Geometry: see drawing. Coordinates: mm, zero at the bounding-box minimum. A direction names the side the tool comes from. Give positions to 0.01 mm unless a question says otherwise; leave off trailing zeros. Order: outer loops, then holes, each group sorted by start corner. A loop starts at its lowest first (then second) coordinate and runs counter-clockwise, first axis right, second up. Notation, with made-up numbers: (82, 55.5) - (93, 55.5) arc R31 cw to (93, 87.5) - close; hole circle Ø11 at (-29.75, 64.25). An arc over 180 degrees is marked (long way). Put each result on its own line as item: value. Start each with the question number.
1. First-contact query: P1, Ø5.5, axis at y = 5, z = 32, coming from the -X side; P2, Ø5, axis at x = 19.85, z = 14, coming from the -Y side; P3, Ø3, axis at x = 52.25, y = 4.9, coming from the +Z side; P4, Ø10, axis at y = 14.5, z = 17.5, coming from the +X side. Flat tips, straight axial feed; report the tip coordinate or a pass-through.
2. Section B-B on x = 52.25. Return the cut outline in (y, z).
3. Section D-D on z = 14. Return the cut outline in (x, y), plus the area to 3 significant figures.
4. Set-up query: the marked faces 4, 5, 6, 7 and 8. Return all of +Z, -Z, +X, -X, +Y, -Y with unobstructed straight access to the full face (end or side cutting, diameter ignored); none if empty.
5. Section C-C on x = 19.85. Return the cut outline in (y, z), plus the area to 3 significant figures.
6. Ray query, line 1 along Y through (x, z) = (52.25, 27.75); line 2 along Z through (x, y) = (19.85, 14.75); line 3 along Z through (x, y) = (45, 6.75). Return the intervals inside material, ascending. Write a range as from..to.
7. Section A-A on y = 14.9. Return the cut outline in (x, z), plus the area to 3 significant figures.
8. Mould query, pull axis Z, two halves, no side actions, for the marked faces 1, 2 and 3. Classes: pulls with the +Z half, pulls with the -Z half, needs draft (parallel to the pull), parting line crosses it, or undercut.
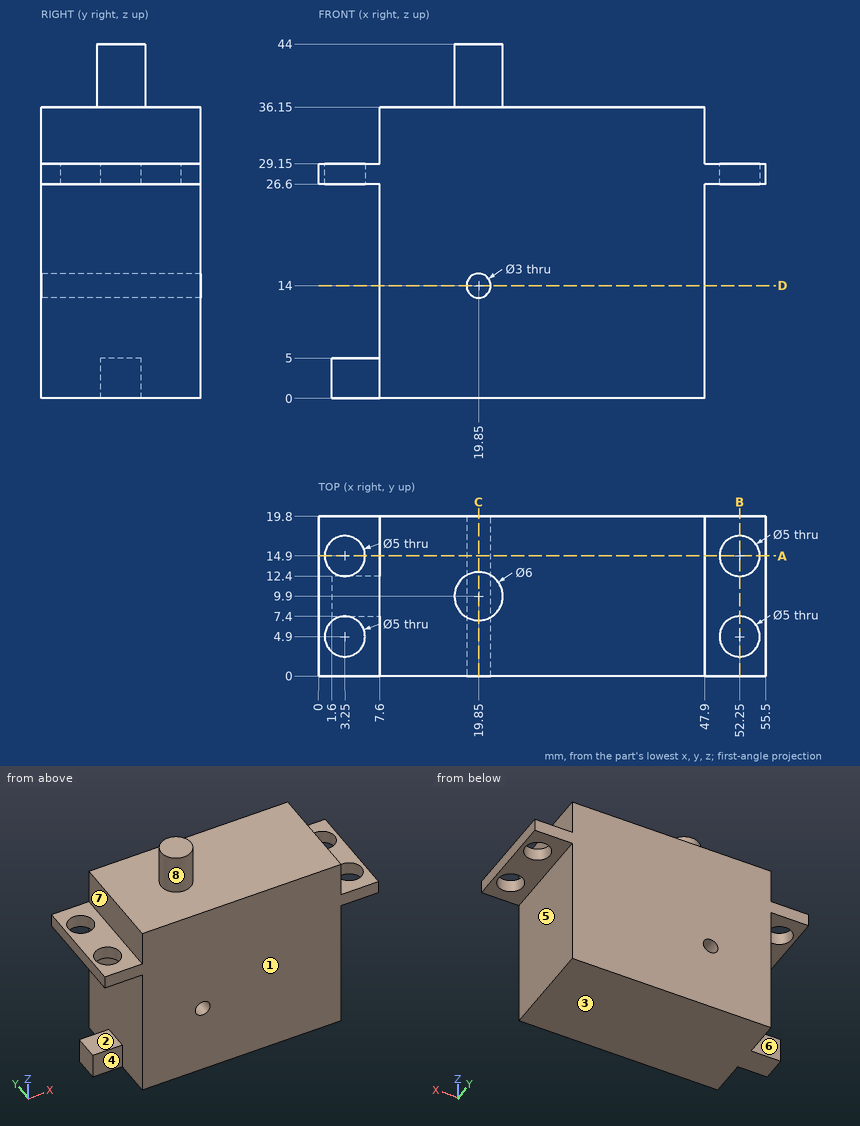
Resolved:
1. P1: x = 7.6
1. P2: y = 0
1. P3: through
1. P4: x = 47.9
2. outline: (0, 26.6) - (2.4, 26.6) - (2.4, 29.15) - (0, 29.15) - close; (7.4, 26.6) - (12.4, 26.6) - (12.4, 29.15) - (7.4, 29.15) - close; (17.4, 26.6) - (19.8, 26.6) - (19.8, 29.15) - (17.4, 29.15) - close
3. outline: (7.6, 0) - (18.35, 0) - (18.35, 19.8) - (7.6, 19.8) - close; (21.35, 0) - (47.9, 0) - (47.9, 19.8) - (21.35, 19.8) - close
3. area: 739 mm^2
4. face 4: -Z, -X, -Y
4. face 5: -Z, +X, +Y, -Y
4. face 6: -Z, -X, +Y
4. face 7: +Z, -X, +Y, -Y
4. face 8: +Z
5. outline: (0, 0) - (19.8, 0) - (19.8, 12.5) - (0, 12.5) - close; (0, 15.5) - (19.8, 15.5) - (19.8, 36.15) - (12.9, 36.15) - (12.9, 44) - (6.9, 44) - (6.9, 36.15) - (0, 36.15) - close
5. area: 703 mm^2
6. line 1: 0..2.4, 7.4..12.4, 17.4..19.8
6. line 2: 0..12.5, 15.5..36.15
6. line 3: 0..36.15
7. outline: (0, 26.6) - (0.75, 26.6) - (0.75, 29.15) - (0, 29.15) - close; (5.75, 26.6) - (7.6, 26.6) - (7.6, 0) - (47.9, 0) - (47.9, 26.6) - (49.75, 26.6) - (49.75, 29.15) - (47.9, 29.15) - (47.9, 36.15) - (7.6, 36.15) - (7.6, 29.15) - (5.75, 29.15) - close; (54.75, 26.6) - (55.5, 26.6) - (55.5, 29.15) - (54.75, 29.15) - close; hole circle Ø3 at (19.85, 14)
7. area: 1,460 mm^2
8. face 1: needs draft
8. face 2: undercut
8. face 3: pulls with the -Z half
